The listing builds one solid part. Answer for the finished solid, in the listing's coordinates (mm). A direction names the side the tool comes from. Give positions to 0.01 mm unless a question says otherwise; leave off trailing zeros. Order: outer loops, then holes, each group sorted by start corner. A loop starts at its lowest first (then second) coordinate and runs counter-clockwise, first axis right, second up. Notation, with made-up numbers: (-40, 82) - (10, 82) arc R15 ccw to (10, 109) - close; hole circle Ø6 at (12.25, 26). An arc over 180 degrees is marked (long way). Answer in a Markdown table with one row per item.
from build123d import *

# Parameters (mm, degrees)
SKETCH1_W             = 40.2336
SKETCH1_H             = 22.0218
BOSS_EXTRUDE1_DEPTH   = 3.3
FILLET1_R             = 2.5908
SKETCH3_W             = 38.608
SKETCH3_H             = 21.209
CUT_EXTRUDE1_DEPTH    = 0.5588
FILLET2_R             = 1.778
SKETCH4_R             = 1.375
CUT_EXTRUDE2_DEPTH    = 24.096314392
SKETCH5_R             = 3.045
CUT_EXTRUDE3_DEPTH    = 2.25
SKETCH6_W             = 2.54
SKETCH6_H             = 10.16
CUT_EXTRUDE4_DEPTH    = 1.27
FILLET3_R             = 1
FILLET3_OF_MIRROR3_R  = 1
BOSS_EXTRUDE2_DEPTH   = 20.8
SKETCH9_W             = 38.608
SKETCH9_H             = 20
BOSS_EXTRUDE3_DEPTH   = 0.2
MIRROR4_OUTLINE_R     = 3.045
MIRROR4_DEPTH         = 2.7412
MIRROR4_2_DEPTH       = 1.4712
MIRROR4_START         = 2.25
MIRROR4_3_OUTLINE_R   = 3.045
MIRROR4_3_OUTLINE_R_2 = 1.375
MIRROR4_3_DEPTH       = 0.4912
MIRROR4_START_2       = 2.7412
MIRROR4_4_DEPTH       = 0.5588


# Read off the part's stored shape, not the designer's step: Mirror4
with BuildPart() as part:
    # Sketch1 → Boss-Extrude1 (new body)
    with BuildSketch(Plane(origin=(0, 0, 0), x_dir=(1, 0, 0), z_dir=(0, 1, 0))):
        Rectangle(SKETCH1_W, SKETCH1_H)
    extrude(amount=BOSS_EXTRUDE1_DEPTH)

    # Fillet1
    fillet1_edges = [part.edges().sort_by_distance(p)[0] for p in [
        (-20.1168, 1.65, -11.0109),
        (20.1168, 1.65, -11.0109),
    ]]
    fillet(fillet1_edges, radius=FILLET1_R)

    # Sketch3 → Cut-Extrude1 (cut)
    with BuildSketch(Plane(origin=(0, 3.3, 0), x_dir=(1, 0, 0), z_dir=(0, 1, 0))):
        with Locations((0, -0.4064)):
            Rectangle(SKETCH3_W, SKETCH3_H)
    extrude(amount=-CUT_EXTRUDE1_DEPTH, mode=Mode.SUBTRACT)

    # Fillet2
    fillet2_edges = [part.edges().sort_by_distance(p)[0] for p in [
        (19.304, 3.0206, -10.1981),
        (-19.304, 3.0206, -10.1981),
    ]]
    fillet(fillet2_edges, radius=FILLET2_R)

    # Sketch4 → Cut-Extrude2 (cut, through all)
    with BuildSketch(Plane(origin=(0, 2.7412, 0), x_dir=(1, 0, 0), z_dir=(0, 1, 0))):
        with Locations(Location((-6.35, 6.7691, 0), (0, 0, 270))):
            Circle(SKETCH4_R)
        with Locations(Location((-15.24, -4.0259, 0), (0, 0, 270))):
            Circle(SKETCH4_R)
    cut_extrude2 = extrude(amount=-CUT_EXTRUDE2_DEPTH, mode=Mode.SUBTRACT)

    # Mirror1: Cut-Extrude2 across plane
    add(cut_extrude2.mirror(Plane(origin=(0, 0, 0), x_dir=(0, 0, 1), z_dir=(1, 0, 0))), mode=Mode.SUBTRACT)

    # Sketch5 → Cut-Extrude3 (cut)
    with BuildSketch(Plane.XZ):
        with Locations(Location((-15.24, 4.0259, 0), (0, 0, 270))):
            Circle(SKETCH5_R)
        with Locations(Location((-6.35, -6.7691, 0), (0, 0, 270))):
            Circle(SKETCH5_R)
    cut_extrude3 = extrude(amount=-CUT_EXTRUDE3_DEPTH, mode=Mode.SUBTRACT)

    # Mirror2: Cut-Extrude3 across plane
    add(cut_extrude3.mirror(Plane(origin=(0, 0, 0), x_dir=(0, 0, 1), z_dir=(1, 0, 0))), mode=Mode.SUBTRACT)

    # Sketch6 → Cut-Extrude4 (cut)
    with BuildSketch(Plane(origin=(0, 2.7412, 0), x_dir=(1, 0, 0), z_dir=(0, 1, 0))):
        with Locations((-11.43, 3.9751)):
            Rectangle(SKETCH6_W, SKETCH6_H)
    cut_extrude4 = extrude(amount=-CUT_EXTRUDE4_DEPTH, mode=Mode.SUBTRACT)

    # Fillet3
    fillet3_edges = [part.edges().sort_by_distance(p)[0] for p in [
        (-10.16, 2.1062, -9.0551),
        (-10.16, 2.1062, 1.1049),
        (-12.7, 2.1062, 1.1049),
        (-12.7, 2.1062, -9.0551),
    ]]
    fillet(fillet3_edges, radius=FILLET3_R)

    # Mirror3: Cut-Extrude4 across plane
    add(cut_extrude4.mirror(Plane(origin=(0, 0, 0), x_dir=(0, 0, 1), z_dir=(1, 0, 0))), mode=Mode.SUBTRACT)

    # Fillet3 of Mirror3
    fillet3_of_mirror3_edges = [part.edges().sort_by_distance(p)[0] for p in [
        (10.16, 2.1062, -9.0551),
        (10.16, 2.1062, 1.1049),
        (12.7, 2.1062, 1.1049),
        (12.7, 2.1062, -9.0551),
    ]]
    fillet(fillet3_of_mirror3_edges, radius=FILLET3_OF_MIRROR3_R)

    # Sketch8 → Boss-Extrude2 (add)
    with BuildSketch(Plane.XY.offset(11.0109)):
        Polygon((-20.1168, 0), (-20.1168, 3.3), (-19.304, 3.3), (-19.304, 2.7412), (19.304, 2.7412), (19.304, 3.3), (20.1168, 3.3), (20.1168, 0), align=None)
    extrude(amount=BOSS_EXTRUDE2_DEPTH)

    # Sketch9 → Boss-Extrude3 (add)
    with BuildSketch(Plane(origin=(0, 2.7412, 0), x_dir=(1, 0, 0), z_dir=(0, 1, 0))):
        with Locations((0, -21.4109)):
            Rectangle(SKETCH9_W, SKETCH9_H)
    extrude(amount=BOSS_EXTRUDE3_DEPTH)

    # Mirror4 outline → Mirror4 (add)
    with BuildSketch(Plane(origin=(0, 0, 0), x_dir=(1, 0, 0), z_dir=(0, 1, 0))):
        with BuildLine():
            Line((-20.1168, -31.8109), (-20.1168, -51.241899868))
            ThreePointArc((-20.1168, -51.241899868), (-19.357972249, -53.073872117), (-17.526, -53.832699868))
            Line((-17.526, -53.832699868), (17.526, -53.832699868))
            ThreePointArc((17.526, -53.832699868), (19.357972249, -53.073872117), (20.1168, -51.241899868))
            Line((20.1168, -51.241899868), (20.1168, -31.8109))
            Line((20.1168, -31.8109), (-20.1168, -31.8109))
        make_face()
        with Locations((-6.35, -49.590899868)):
            Circle(MIRROR4_OUTLINE_R, mode=Mode.SUBTRACT)
        with BuildLine():
            ThreePointArc((-11.16, -41.716899868), (-10.452893219, -42.009793087), (-10.16, -42.716899868))
            Line((-10.16, -42.716899868), (-10.16, -50.876899868))
            ThreePointArc((-10.16, -50.876899868), (-10.452893219, -51.584006649), (-11.16, -51.876899868))
            Line((-11.16, -51.876899868), (-11.7, -51.876899868))
            ThreePointArc((-11.7, -51.876899868), (-12.407106781, -51.584006649), (-12.7, -50.876899868))
            Line((-12.7, -50.876899868), (-12.7, -42.716899868))
            ThreePointArc((-12.7, -42.716899868), (-12.407106781, -42.009793087), (-11.7, -41.716899868))
            Line((-11.7, -41.716899868), (-11.16, -41.716899868))
        make_face(mode=Mode.SUBTRACT)
        with Locations((6.35, -49.590899868)):
            Circle(MIRROR4_OUTLINE_R, mode=Mode.SUBTRACT)
        with BuildLine():
            Line((10.16, -50.876899868), (10.16, -42.716899868))
            ThreePointArc((10.16, -42.716899868), (10.452893219, -42.009793087), (11.16, -41.716899868))
            Line((11.16, -41.716899868), (11.7, -41.716899868))
            ThreePointArc((11.7, -41.716899868), (12.407106781, -42.009793087), (12.7, -42.716899868))
            Line((12.7, -42.716899868), (12.7, -50.876899868))
            ThreePointArc((12.7, -50.876899868), (12.407106781, -51.584006649), (11.7, -51.876899868))
            Line((11.7, -51.876899868), (11.16, -51.876899868))
            ThreePointArc((11.16, -51.876899868), (10.452893219, -51.584006649), (10.16, -50.876899868))
        make_face(mode=Mode.SUBTRACT)
        with Locations((-15.24, -38.795899868)):
            Circle(MIRROR4_OUTLINE_R, mode=Mode.SUBTRACT)
        with Locations((15.24, -38.795899868)):
            Circle(MIRROR4_OUTLINE_R, mode=Mode.SUBTRACT)
    extrude(amount=MIRROR4_DEPTH)

    # Mirror4 2 outline → Mirror4 2 (add)
    with BuildSketch(Plane(origin=(0, 0, 0), x_dir=(1, 0, 0), z_dir=(0, 1, 0))):
        with BuildLine():
            Line((-10.16, -50.876899868), (-10.16, -42.716899868))
            ThreePointArc((-10.16, -42.716899868), (-10.452893219, -42.009793087), (-11.16, -41.716899868))
            Line((-11.16, -41.716899868), (-11.7, -41.716899868))
            ThreePointArc((-11.7, -41.716899868), (-12.407106781, -42.009793087), (-12.7, -42.716899868))
            Line((-12.7, -42.716899868), (-12.7, -50.876899868))
            ThreePointArc((-12.7, -50.876899868), (-12.407106781, -51.584006649), (-11.7, -51.876899868))
            Line((-11.7, -51.876899868), (-11.16, -51.876899868))
            ThreePointArc((-11.16, -51.876899868), (-10.452893219, -51.584006649), (-10.16, -50.876899868))
        make_face()
        with BuildLine():
            ThreePointArc((11.16, -41.716899868), (10.452893219, -42.009793087), (10.16, -42.716899868))
            Line((10.16, -42.716899868), (10.16, -50.876899868))
            ThreePointArc((10.16, -50.876899868), (10.452893219, -51.584006649), (11.16, -51.876899868))
            Line((11.16, -51.876899868), (11.7, -51.876899868))
            ThreePointArc((11.7, -51.876899868), (12.407106781, -51.584006649), (12.7, -50.876899868))
            Line((12.7, -50.876899868), (12.7, -42.716899868))
            ThreePointArc((12.7, -42.716899868), (12.407106781, -42.009793087), (11.7, -41.716899868))
            Line((11.7, -41.716899868), (11.16, -41.716899868))
        make_face()
    extrude(amount=MIRROR4_2_DEPTH)

    # Mirror4 3 outline → Mirror4 3 (add)
    # profile 1 of 4: a face of its own
    with BuildSketch(Plane(origin=(0, 0, 0), x_dir=(1, 0, 0), z_dir=(0, 1, 0)).offset(MIRROR4_START)):
        with Locations((-6.35, -49.590899868)):
            Circle(MIRROR4_3_OUTLINE_R)
        with Locations((-6.35, -49.590899868)):
            Circle(MIRROR4_3_OUTLINE_R_2, mode=Mode.SUBTRACT)
    # profile 2 of 4: a face of its own
    with BuildSketch(Plane(origin=(0, 0, 0), x_dir=(1, 0, 0), z_dir=(0, 1, 0)).offset(MIRROR4_START)):
        with Locations((-15.24, -38.795899868)):
            Circle(MIRROR4_3_OUTLINE_R)
        with Locations((-15.24, -38.795899868)):
            Circle(MIRROR4_3_OUTLINE_R_2, mode=Mode.SUBTRACT)
    # profile 3 of 4: a face of its own
    with BuildSketch(Plane(origin=(0, 0, 0), x_dir=(1, 0, 0), z_dir=(0, 1, 0)).offset(MIRROR4_START)):
        with Locations((6.35, -49.590899868)):
            Circle(MIRROR4_3_OUTLINE_R)
        with Locations((6.35, -49.590899868)):
            Circle(MIRROR4_3_OUTLINE_R_2, mode=Mode.SUBTRACT)
    # profile 4 of 4: a face of its own
    with BuildSketch(Plane(origin=(0, 0, 0), x_dir=(1, 0, 0), z_dir=(0, 1, 0)).offset(MIRROR4_START)):
        with Locations((15.24, -38.795899868)):
            Circle(MIRROR4_3_OUTLINE_R)
        with Locations((15.24, -38.795899868)):
            Circle(MIRROR4_3_OUTLINE_R_2, mode=Mode.SUBTRACT)
    extrude(amount=MIRROR4_3_DEPTH)

    # Mirror4 4 outline → Mirror4 4 (add)
    with BuildSketch(Plane(origin=(0, 0, 0), x_dir=(1, 0, 0), z_dir=(0, 1, 0)).offset(MIRROR4_START_2)):
        with BuildLine():
            Line((19.304, -31.8109), (19.304, -51.241899868))
            ThreePointArc((19.304, -51.241899868), (18.783235857, -52.499135725), (17.526, -53.019899868))
            Line((17.526, -53.019899868), (-17.526, -53.019899868))
            ThreePointArc((-17.526, -53.019899868), (-18.783235857, -52.499135725), (-19.304, -51.241899868))
            Line((-19.304, -51.241899868), (-19.304, -31.8109))
            Line((-19.304, -31.8109), (-20.1168, -31.8109))
            Line((-20.1168, -31.8109), (-20.1168, -51.241899868))
            ThreePointArc((-20.1168, -51.241899868), (-19.357972249, -53.073872117), (-17.526, -53.832699868))
            Line((-17.526, -53.832699868), (17.526, -53.832699868))
            ThreePointArc((17.526, -53.832699868), (19.357972249, -53.073872117), (20.1168, -51.241899868))
            Line((20.1168, -51.241899868), (20.1168, -31.8109))
            Line((20.1168, -31.8109), (19.304, -31.8109))
        make_face()
    extrude(amount=MIRROR4_4_DEPTH)


solid = part.part
Item 1: Find section C-C on z = 26. Write down the section's boundary in (x, y).
Answer block:
| item | result |
|---|---|
| outline | (-20.12, 0) - (20.12, 0) - (20.12, 3.3) - (19.3, 3.3) - (19.3, 2.94) - (-19.3, 2.94) - (-19.3, 3.3) - (-20.12, 3.3) - close |
Item 2: Which of the six approach directions +Z, -Z, +X, -X, +Y, -Y give full straight-line access (tool end or side, diameter ignored) to faces 1 (the face through (19.34, 1.63, 53.09)), 2 (the face through (0, 2.741, 42)), 3 (the face through (-5.435, 1.109, -9.673))?
Answer block:
| item | result |
|---|---|
| face 1 | +Z, +X, +Y, -Y |
| face 2 | +Y |
| face 3 | -Y |
Item 3: Find section B-B on y = 0.7. Count the separate pieces of the cut face and the enclosed holes in it, then the cut area to 3 significant figures.
Answer block:
| item | result |
|---|---|
| separate pieces | 1 |
| enclosed holes | 8 |
| area | 2,370 mm² |
Item 4: Determine the mould class of faces 4 (the face through (-16.253, 2.492, 37.867)), 5 (the face through (-19.38, 1.67, -10.23)), 6 (the face through (0, 2, 53.833)), 7 (the face through (-12.7, 2, 47)) for opening direction X: pulls with the +X half, pulls with the -X half, needs draft (parallel to the pull), parting line crosses it, or undercut.
Answer block:
| item | result |
|---|---|
| face 4 | undercut |
| face 5 | pulls with the -X half |
| face 6 | needs draft |
| face 7 | undercut |
Item 5: Each of these flat-tipped pins is pushed along its axis until it touches: P1, Ø4, axis at x = -8.5, z = 10.5, coming from the +Y side; P2, Ø2, axis at x = -12, z = -5, coming from the +Y side; P3, Ø3, axis at x = -15.24, z = 4.03, coming from the -Y side; P4, Ø2.5, axis at x = -6.35, z = -6.77, coming from the +Y side. Where does it stop, or does it pass through?
Answer block:
| item | result |
|---|---|
| P1 | y = 2.94 |
| P2 | y = 2.74 |
| P3 | y = 2.25 |
| P4 | through |
Item 6: Consider line 1 (Z direction, x = 15.24, y = 2.5); line 2 (Z direction, x = 6.5, y = 1.1); line 3 (X direction, y = 0.3, z = 39). Determine where each line is inside the solid, lowest interval first.
Answer block:
| item | result |
|---|---|
| line 1 | -11.01 to 2.65, 5.4 to 37.42, 40.17 to 53.83 |
| line 2 | -11.01 to -9.81, -3.73 to 46.55, 52.63 to 53.83 |
| line 3 | -20.12 to -18.28, -12.2 to 12.2, 18.28 to 20.12 |
Item 7: Find section A-A on x = -6.35. Write down the section's boundary in (y, z).
Answer block:
| item | result |
|---|---|
| outline | (0, -11.01) - (3.3, -11.01) - (3.3, -10.2) - (2.74, -10.2) - (2.74, -8.14) - (2.25, -8.14) - (2.25, -9.81) - (0, -9.81) - close; (0, -3.72) - (2.25, -3.72) - (2.25, -5.39) - (2.74, -5.39) - (2.74, 11.41) - (2.94, 11.41) - (2.94, 31.41) - (2.74, 31.41) - (2.74, 48.22) - (2.25, 48.22) - (2.25, 46.55) - (0, 46.55) - close; (0, 52.64) - (2.25, 52.64) - (2.25, 50.97) - (2.74, 50.97) - (2.74, 53.02) - (3.3, 53.02) - (3.3, 53.83) - (0, 53.83) - close |
